Read the model definition and answer for the solid it produces. Units are mm, in the model's axes. Coordinates: 2 decimals unless noted, no trailing zeros. Loops run counter-clockwise (first coordinate to the right, second up) from the corner with the lowest first, then second, coordinate; pieces in that order, holes last. Notation, with made-up numbers: (84.5, -39.5) - (116.5, -39.5) arc R31 ccw to (116.5, -9.5) - close; hole circle Ø2 at (-32.75, 4). An arc over 180 degrees is marked (long way). Use one line per item in the form item = value. Start each with the question number.
1) A cutting plane is placed at C-C (x = 999.5). Give the vertices of the cut face in (y, z), and give its area (3 significant figures).
2) A cutting plane is placed at A-A (z = 0). Give the vertices of the cut face in (x, y), and give its area (3 significant figures).
3) Consider line 1 (Y direction, x = -0.1, z = 0); line 2 (Z direction, x = 657, y = -2.25); line 3 (X direction, y = -3, z = -2.5). Determine where each line is inside the solid, lowest interval first.
4) Each of these flat-tipped pins is pushed along its axis until it touches: P1, Ø4, axis at x = 263.5, y = -2.5, coming from the -Z side; P2, Ø1, axis at y = 0, z = 1.5, coming from the +X side; P3, Ø1, axis at x = 445.5, z = 1.5, coming from the -Y side; P4, Ø2, axis at x = 827, z = -3.5, coming from the -Y side. Where does it stop, or does it pass through?
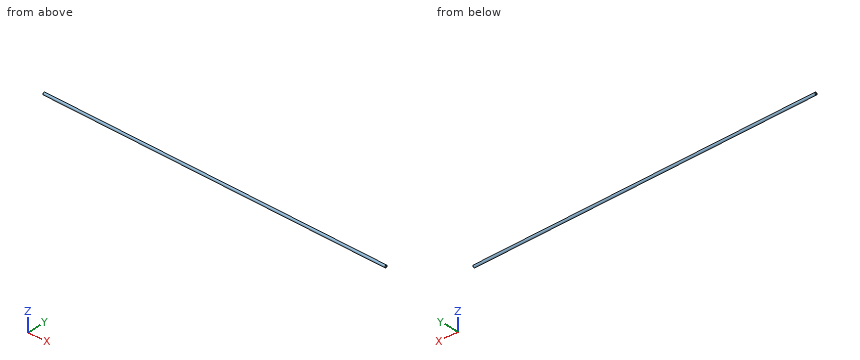
from build123d import *


with BuildPart() as part:
    # Sketch1 → Revolve1 (revolve)
    with BuildSketch(Plane.XY):
        with BuildLine():
            Line((-0.445028708, 3.689878708), (-0.2794, 3.52425))
            Line((-0.2794, 3.52425), (0, 3.52425))
            Line((0, 3.52425), (0.5588, 4.08305))
            Line((0.5588, 4.08305), (1288.2372, 4.08305))
            Line((1288.2372, 4.08305), (1288.796, 3.52425))
            Line((1288.796, 3.52425), (1289.0754, 3.52425))
            Line((1289.0754, 3.52425), (1289.241028708, 3.689878708))
            ThreePointArc((1289.241028708, 3.689878708), (1289.278226147, 3.779681269), (1289.241028708, 3.869483831))
            Line((1289.241028708, 3.869483831), (1288.714881269, 4.395631269))
            ThreePointArc((1288.714881269, 4.395631269), (1288.533593502, 4.516763883), (1288.31975, 4.5593))
            Line((1288.31975, 4.5593), (0.47625, 4.5593))
            ThreePointArc((0.47625, 4.5593), (0.262406498, 4.516763883), (0.081118731, 4.395631269))
            Line((0.081118731, 4.395631269), (-0.445028708, 3.869483831))
            ThreePointArc((-0.445028708, 3.869483831), (-0.482226147, 3.779681269), (-0.445028708, 3.689878708))
        make_face()
    revolve(axis=Axis((1288.796, 0, 0), (-1, 0, 0)))


solid = part.part
Found:
q1.outline = circle Ø9.12 at (0, 0); hole circle Ø8.17 at (0, 0)
q1.area = 12.9 mm^2
q2.outline = (-0.45, -3.87) - (0.08, -4.4) arc R0.56 ccw to (0.48, -4.56) - (1288.32, -4.56) arc R0.56 ccw to (1288.71, -4.4) - (1289.24, -3.87) arc R0.13 ccw to (1289.24, -3.69) - (1289.08, -3.52) - (1288.8, -3.52) - (1288.24, -4.08) - (0.56, -4.08) - (0, -3.52) - (-0.28, -3.52) - (-0.45, -3.69) arc R0.13 ccw to start; (-0.45, 3.69) - (-0.28, 3.52) - (0, 3.52) - (0.56, 4.08) - (1288.24, 4.08) - (1288.8, 3.52) - (1289.08, 3.52) - (1289.24, 3.69) arc R0.13 ccw to (1289.24, 3.87) - (1288.71, 4.4) arc R0.56 ccw to (1288.32, 4.56) - (0.48, 4.56) arc R0.56 ccw to (0.08, 4.4) - (-0.45, 3.87) arc R0.13 ccw to start
q2.area = 1,230 mm^2
q3.line_1 = -4.21 to -3.52, 3.52 to 4.21
q3.line_2 = -3.97 to -3.41, 3.41 to 3.97
q3.line_3 = -0.41 to 0.38, 1288.42 to 1289.21
q4.P1 = -4.53
q4.P2 = through
q4.P3 = -4.45
q4.P4 = -3.81
